```python
from build123d import *

# Parameters (mm, degrees)
CROQUIS1_R              = 1.6
SALIENTE_EXTRUIR1_DEPTH = 3
CROQUIS2_W              = 3
CROQUIS2_H              = 7.298316333
SALIENTE_EXTRUIR2_DEPTH = 9
CROQUIS3_R              = 1.6
CORTAR_EXTRUIR1_DEPTH   = 16
CORTAR_EXTRUIR2_DEPTH   = 1.6
REDONDEO1_R             = 3


with BuildPart() as part:
    # Croquis1 → Saliente-Extruir1 (new body)
    with BuildSketch(Plane.XY):
        with BuildLine():
            ThreePointArc((0.398971354, 4.482278646), (-4.076947647, 1.904861643), (-3.181980515, -3.181980515))
            ThreePointArc((-3.181980515, -3.181980515), (20, -12.784271247), (43.181980515, -3.181980515))
            ThreePointArc((43.181980515, -3.181980515), (44.076947647, 1.904861643), (39.601028646, 4.482278646))
            ThreePointArc((39.601028646, 4.482278646), (20, -5), (0.398971354, 4.482278646))
        make_face()
        Circle(CROQUIS1_R, mode=Mode.SUBTRACT)
        with Locations((40, 0)):
            Circle(CROQUIS1_R, mode=Mode.SUBTRACT)
    extrude(amount=SALIENTE_EXTRUIR1_DEPTH)

    # Croquis2 → Saliente-Extruir2 (add)
    with BuildSketch(Plane.XY.offset(3)):
        with Locations((13.5, -8.144055595)):
            Rectangle(CROQUIS2_W, CROQUIS2_H)
        with Locations((26.5, -8.144055595)):
            Rectangle(CROQUIS2_W, CROQUIS2_H)
    extrude(amount=SALIENTE_EXTRUIR2_DEPTH)

    # Croquis3 → Cortar-Extruir1 (cut)
    with BuildSketch(Plane.ZY.offset(-12)):
        with Locations((8, -8.144897428)):
            Circle(CROQUIS3_R)
    extrude(amount=-CORTAR_EXTRUIR1_DEPTH, mode=Mode.SUBTRACT)

    # Croquis4 → Cortar-Extruir2 (cut)
    with BuildSketch(Plane(origin=(28, 0, 0), x_dir=(0, 0, -1), z_dir=(1, 0, 0))):
        Polygon((-5.401923789, -9.644897428), (-5.401923789, -6.644897428), (-8, -5.144897428), (-10.598076211, -6.644897428), (-10.598076211, -9.644897428), (-8, -11.144897428), align=None)
    extrude(amount=-CORTAR_EXTRUIR2_DEPTH, mode=Mode.SUBTRACT)

    # Redondeo1
    redondeo1_edges = [part.edges().sort_by_distance(p)[0] for p in [
        (13.5, -11.793213761, 12),
        (13.5, -4.494897428, 12),
        (26.5, -4.494897428, 12),
        (26.5, -11.793213761, 12),
    ]]
    fillet(redondeo1_edges, radius=REDONDEO1_R)


solid = part.part
```
Here's how the part is built. I have some questions about the finished solid (model axes, mm). A direction names the side the tool comes from. Give positions to 0.01 mm unless a question says otherwise; leave off trailing zeros. Order: outer loops, then holes, each group sorted by start corner. A loop starts at its lowest first (then second) coordinate and runs counter-clockwise, first axis right, second up. Notation, with made-up numbers: M 0,28 L 26,28 A17 ccw 26,58 Z; hole C 20.5,83 d9. An arc over 180 degrees is marked long. Use a Markdown table: item, result. Add a question column.
1. Suppose I cut it at B-B (x = 1). List the corners of the cut face in (y, z) for me.
2. Suppose I cut it at D-D (y = 2.25). List the corners of the cut face in (x, z) for me, and give its area (3 significant figures).
3. Suppose I cut it at C-C (z = 7.5). List the corners of the cut face in (x, y) for me, and give its area (3 significant figures).
4. Suppose I cut it at A-A (y = 0). List the corners of the cut face in (x, z) for me, and give its area (3 significant figures).
5. I need wall thicknesses on probe 1 along X at (y, z) = (-0.5, 2.75); probe 2 along X at (y, z) = (-6.75, 9); probe 3 along Z at (x, y) = (11, -6.5). Which ranges of each line are inside material? Lowest first, please. Write a range as from..to.
6. On a 3-axis mill with a long thin cutter (end or side, diameter ignored), from which of +Z, -Z, +X, -X, +Y, -Y can I reach the whole of each face in a straight line? I mean faces 1 (the flat face through (28, -7, 5)), 2 (the flat face through (27.211, -10.405, 6.719)), 3 (the flat face through (26, -11.793, 6)), 4 (the flat face through (26, -4.495, 6)), 5 (the flat face through (15, -7, 6)). Say none if no direction works.
7. If we mould it in two halves opening along Y, with no side actions, what happens to faces 6 (the flat face through (27.211, -10.384, 9.317)), 7 (the flat face through (13, -8, 12)), 8 (the flat face through (27.211, -5.905, 6.683)), 9 (the cylindrical face through (44.11, 1.83, 1.48))? For each: +Y half, -Y half, draft (parallel to the pull), parting line (faces both ways), or undercut.
8. For pin 1 Ø2.5 at (y, z) = (-8.5, 7.5) entering from +X; pin 2 Ø3.5 at (y, z) = (-8.14, 8) entering from -X; pin 3 Ø5 at (x, y) = (40, 0) entering from +Z; pin 4 Ø2.5 at (x, y) = (0, 0) entering from +Z, each with a flat end and sliding along its axis, tell me the tip position at first contact or that it passes through.
Results list:
| question | item | result |
|---|---|---|
| 1 | outline | M -6.72,0 L -1.25,0 L -1.25,3 L -6.72,3 Z; M 1.25,0 L 3.75,0 L 3.75,3 L 1.25,3 Z |
| 2 | outline | M -3.9,0 L 2.39,0 L 2.39,3 L -3.9,3 Z; M 37.61,0 L 43.9,0 L 43.9,3 L 37.61,3 Z |
| 2 | area | 37.8 mm² |
| 3 | outline | M 12,-11.79 L 15,-11.79 L 15,-9.66 L 12,-9.66 Z; M 12,-6.63 L 15,-6.63 L 15,-4.49 L 12,-4.49 Z; M 25,-11.79 L 28,-11.79 L 28,-10.86 L 26.4,-10.86 L 26.4,-9.66 L 25,-9.66 Z; M 25,-6.63 L 26.4,-6.63 L 26.4,-5.43 L 28,-5.43 L 28,-4.49 L 25,-4.49 Z |
| 3 | area | 21.7 mm² |
| 4 | outline | M -4.5,0 L -1.6,0 L -1.6,3 L -4.5,3 Z; M 1.6,0 L 5,0 L 5,3 L 1.6,3 Z; M 35,0 L 38.4,0 L 38.4,3 L 35,3 Z; M 41.6,0 L 44.5,0 L 44.5,3 L 41.6,3 Z |
| 4 | area | 37.8 mm² |
| 5 | probe 1 | x = -4.47..-1.52, 1.52..5.69, 34.31..38.48, 41.52..44.47 |
| 5 | probe 2 | x = 12..15, 25..26.4 |
| 5 | probe 3 | z = 0..3 |
| 6 | face 1 | +Z, +X, +Y, -Y |
| 6 | face 2 | +X |
| 6 | face 3 | +Z, +X, -X, -Y |
| 6 | face 4 | +Z, +X, -X, +Y |
| 6 | face 5 | +Z, +Y, -Y |
| 7 | face 6 | undercut |
| 7 | face 7 | draft |
| 7 | face 8 | undercut |
| 7 | face 9 | parting line |
| 8 | pin 1 | stops at x = 26.4 |
| 8 | pin 2 | stops at x = 12 |
| 8 | pin 3 | stops at z = 3 |
| 8 | pin 4 | passes through |
